Autodesk Inventor part; units mm, degrees
ref_plane "YZ Plane" through (0, 0, 0) normal (1, 0, 0) x (0, 1, 0)
ref_plane "XZ Plane" through (0, 0, 0) normal (0, 1, 0) x (-1, 0, 0)
ref_plane "XY Plane" through (0, 0, 0) normal (0, 0, 1) x (1, 0, 0)
sketch "Sketch1" plane through (0, 0, 0) normal (0, 0, 1) x (1, 0, 0)
  circle A0 centre (0, 0) radius 5.1
  circle A1 centre (0, 0) radius 4
  dimension "d0" = 10.2
  dimension "d1" = 8
extrude "Extrusion1" add sketch "Sketch1" along normal blind 10
sketch "Sketch2" plane through (0, 0, 0) normal (0, 0, -1) x (-1, 0, 0)
  circle A0 centre (0, 0) radius 4
  circle A1 centre (0, 0) radius 11
  dimension "d4" = 8
  dimension "d5" = 22
extrude "Extrusion2" add sketch "Sketch2" along normal blind 3.5
sketch "Sketch3" plane through (0, 0, -3.5) normal (0, 0, -1) x (-1, 0, 0)
  circle A0 centre (0, 0) radius 4
  circle A1 centre (0, 0) radius 5.1
  dimension "d8" = 8
  dimension "d9" = 10.2
extrude "Extrusion3" add sketch "Sketch3" along normal blind 1.5
sketch "Sketch4" plane through (0, 0, -3.5) normal (0, 0, -1) x (-1, 0, 0)
  circle A0 centre (0, 0) radius 8
  circle A1 centre (0, -8) radius 1.75
  circle A2 centre (8, 0) radius 1.75
  circle A3 centre (0, 8) radius 1.75
  circle A4 centre (-8, 0) radius 1.75
  dimension "d12" = 16
  dimension "d13" = 3.5
  dimension "d16" = 360
extrude "Extrusion4" cut sketch "Sketch4" against normal blind 3.5 contours A0 A2 | A0 A2 | A3 A0 | A0 A3 | A1 A0 | A0 A1 | A4 A0 | A0 A4
properties part number "TUERCA DE HUSILLO"
Verification items for the finished model (mm, model axes). A direction names the side the tool comes from. Coordinates: 2 decimals unless noted, no trailing zeros. Order: outer loops, then holes, each group sorted by start corner. A loop starts at its lowest first (then second) coordinate and runs counter-clockwise, first axis right, second up. Notation, with made-up numbers: M 51.5,17 L 56.5,17 A23 ccw 56.5,55 Z; hole C 35,26 d6. An arc over 180 degrees is marked long. One line per item, written item: value. Start each with the question number.
Item 1: Gauge pin test, flat ends, axial feed: pin 1 (8 mm diameter, centred on x = -4.5, z = 1, fed in from -Y); pin 2 (8 mm diameter, centred on y = -7, z = 5, fed in from +X); pin 3 (1 mm diameter, centred on x = 8, y = 5.5, fed in from +Z). Record the tip position at first contact, or that the pin passes through.
Item 2: Mould release check, pull along X, two halves, no side actions. Record for faces 4 (the flat face through (-3, -3, 10)), 5 (the cylindrical face through (2.38, 10.74, -1.73)), 6 (the cylindrical face through (-9.669, 0.526, -1.774)), 7 (the cylindrical face through (6.331, 0.526, -1.774)): released by +X, released by -X, zero draft, split by the parting line, or undercut.
Item 3: Sectioned sample at B-B (z = -3). Enter the section's corners in (x, y), then the cut area to 3 significant figures.
Item 4: Sectioned sample at A-A (x = 0). Enter the section's corners in (y, z), then the cut area to 3 significant figures.
Item 5: Sectioned sample at D-D (y = -1). Enter the section's corners in (x, z), then the cut area to 3 significant figures.
Item 6: Scan lines: probe 1 along Y at (x, z) = (0, -2.2); probe 2 along Y at (x, z) = (0, -4); probe 3 along X at (y, z) = (1.75, 6). Record each from-to range of solid material in increasing order.
Item 7: Sectioned sample at C-C (x = 8.75). Enter the section's corners in (y, z), then the cut area to 3 significant figures.
Item 8: Access from +Z, -Z, +X, -X, +Y, -Y to the whole of each face (thin tool, end or side, straight path). Record for faces 1 (the flat face through (-5, -2, 0)), 2 (the flat face through (3, -3, -5)), 3 (the cylindrical face through (-2.4, 4.5, -4.2)).
Conclusion:
1. pin 1: stops at y = -10.98
1. pin 2: stops at x = 4.12
1. pin 3: stops at z = 0
2. face 4: zero draft
2. face 5: split by the parting line
2. face 6: undercut
2. face 7: undercut
3. outline: C 0,0 d22; hole C -8,0 d3.5; hole C 0,0 d8; hole C 0,-8 d3.5; hole C 0,8 d3.5; hole C 8,0 d3.5
3. area: 291 mm^2
4. outline: M -11,-3.5 L -9.75,-3.5 L -9.75,0 L -11,0 Z; M -6.25,-3.5 L -5.1,-3.5 L -5.1,-5 L -4,-5 L -4,10 L -5.1,10 L -5.1,0 L -6.25,0 Z; M 4,-5 L 5.1,-5 L 5.1,-3.5 L 6.25,-3.5 L 6.25,0 L 5.1,0 L 5.1,10 L 4,10 Z; M 9.75,-3.5 L 11,-3.5 L 11,0 L 9.75,0 Z
4. area: 49.8 mm^2
5. outline: M -10.95,-3.5 L -9.44,-3.5 L -9.44,0 L -10.95,0 Z; M -6.56,-3.5 L -5,-3.5 L -5,-5 L -3.87,-5 L -3.87,10 L -5,10 L -5,0 L -6.56,0 Z; M 3.87,-5 L 5,-5 L 5,-3.5 L 6.56,-3.5 L 6.56,0 L 5,0 L 5,10 L 3.87,10 Z; M 9.44,-3.5 L 10.95,-3.5 L 10.95,0 L 9.44,0 Z
5. area: 55.4 mm^2
6. probe 1: y = -11 to -9.75, -6.25 to -4, 4 to 6.25, 9.75 to 11
6. probe 2: y = -5.1 to -4, 4 to 5.1
6. probe 3: x = -4.79 to -3.6, 3.6 to 4.79
7. outline: M -6.67,-3.5 L -1.58,-3.5 L -1.58,0 L -6.67,0 Z; M 1.58,-3.5 L 6.67,-3.5 L 6.67,0 L 1.58,0 Z
7. area: 35.6 mm^2
8. face 1: +Z
8. face 2: -Z, +X, -X, +Y, -Y
8. face 3: -Z
